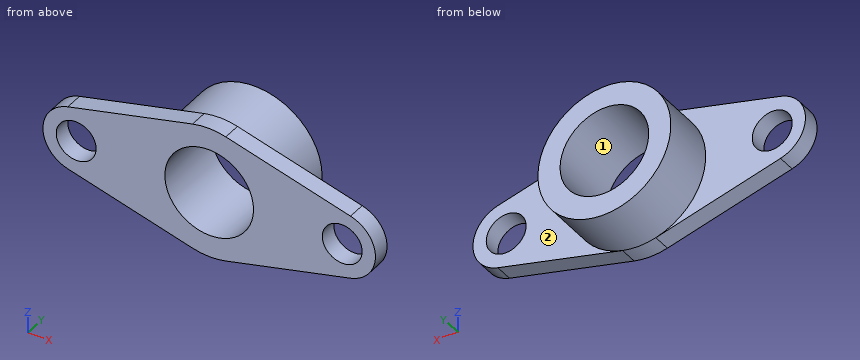
from build123d import *

# Parameters (mm, degrees)
SKETCH2_R           = 2.25
SKETCH2_R_2         = 5
BOSS_EXTRUDE2_DEPTH = 2
SKETCH3_R           = 7.5
SKETCH3_R_2         = 5
BOSS_EXTRUDE3_DEPTH = 6


with BuildPart() as part:
    # Sketch2 → Boss-Extrude2 (new body)
    with BuildSketch(Plane(origin=(0, 0, 0), x_dir=(1, 0, 0), z_dir=(0, 1, 0))):
        with BuildLine():
            Line((-1.875, 7.261843774), (-15.9375, 3.630921887))
            ThreePointArc((-15.9375, 3.630921887), (-18.75, 0), (-15.9375, -3.630921887))
            Line((-15.9375, -3.630921887), (-1.875, -7.261843774))
            ThreePointArc((-1.875, -7.261843774), (0, -7.5), (1.875, -7.261843774))
            Line((1.875, -7.261843774), (15.9375, -3.630921887))
            ThreePointArc((15.9375, -3.630921887), (18.75, 0), (15.9375, 3.630921887))
            Line((15.9375, 3.630921887), (1.875, 7.261843774))
            ThreePointArc((1.875, 7.261843774), (0, 7.5), (-1.875, 7.261843774))
        make_face()
        with Locations((-15, 0)):
            Circle(SKETCH2_R, mode=Mode.SUBTRACT)
        Circle(SKETCH2_R_2, mode=Mode.SUBTRACT)
        with Locations((15, 0)):
            Circle(SKETCH2_R, mode=Mode.SUBTRACT)
    extrude(amount=BOSS_EXTRUDE2_DEPTH)

    # Sketch3 → Boss-Extrude3 (add)
    with BuildSketch(Plane(origin=(0, 2, 0), x_dir=(1, 0, 0), z_dir=(0, 1, 0))):
        Circle(SKETCH3_R)
        Circle(SKETCH3_R_2, mode=Mode.SUBTRACT)
    extrude(amount=BOSS_EXTRUDE3_DEPTH)


solid = part.part
Verification items for the finished model (mm, model axes). Face numbers are marked on the shaded views. Round coordinates to 2 decimals unless told otherwise and drop trailing zeros. Loops run counter-clockwise (first coordinate to the right, second up) from the corner with the lowest first, then second, coordinate; pieces in that order, holes last. Notation, with made-up numbers: (48, 43.25) - (95, 43.25) arc R15 cw to (95, 52.25) - close; hole circle Ø4 at (53.25, -25). An arc over 180 degrees is marked (long way). Use a Markdown table: item, result. Add a question column.
1. Section check A-A, the plane z = 0. Record the boundary of the cut face in (x, y), plus the area to 3 significant figures.
2. Gauge pin test, flat ends, axial feed: pin 1 (2 mm diameter, centred on x = -4.5, y = 4.5, fed in from -Z); pin 2 (2 mm diameter, centred on x = 14, z = -1.5, fed in from +Y). Record the tip position at first contact, or that the pin passes through.
3. Thickness scan on probe 1 along X at (y, z) = (0.75, -1.25); probe 2 along Z at (x, y) = (0, 4.75); probe 3 along X at (y, z) = (7, -3.75). Record the ranges inside material, lowest first. Write a range as [from, to].
4. Release check for a two-part mould opening along X. For the marked faces 1 and 2 record: released by +X, released by -X, zero draft, split by the parting line, or undercut.
5. Section check C-C, the plane x = 0. Record the boundary of the cut face in (y, z).
6. Section check D-D, the plane z = -3. Record the boundary of the cut face in (x, y), plus the area to 3 significant figures.
7. Section check B-B, the plane y = 1.5. Give the number of separate pieces and of enclosed holes in the cut face, plus the area to 3 significant figures.
Checks:
| question | item | result |
|---|---|---|
| 1 | outline | (-18.75, 0) - (-17.25, 0) - (-17.25, 2) - (-18.75, 2) - close; (-12.75, 0) - (-5, 0) - (-5, 8) - (-7.5, 8) - (-7.5, 2) - (-12.75, 2) - close; (5, 0) - (12.75, 0) - (12.75, 2) - (7.5, 2) - (7.5, 8) - (5, 8) - close; (17.25, 0) - (18.75, 0) - (18.75, 2) - (17.25, 2) - close |
| 1 | area | 67.0 mm^2 |
| 2 | pin 1 | stops at z = -6.63 |
| 2 | pin 2 | stops at y = 2 |
| 3 | probe 1 | x = [-18.54, -16.87], [-13.13, -4.84], [4.84, 13.13], [16.87, 18.54] |
| 3 | probe 2 | z = [-7.5, -5], [5, 7.5] |
| 3 | probe 3 | x = [-6.5, -3.31], [3.31, 6.5] |
| 4 | face 1 | undercut |
| 4 | face 2 | zero draft |
| 5 | outline | (0, -7.5) - (8, -7.5) - (8, -5) - (0, -5) - close; (0, 5) - (8, 5) - (8, 7.5) - (0, 7.5) - close |
| 6 | outline | (-17.25, 0) - (-4, 0) - (-4, 8) - (-6.87, 8) - (-6.87, 2) - (-17.25, 2) - close; (4, 0) - (17.25, 0) - (17.25, 2) - (6.87, 2) - (6.87, 8) - (4, 8) - close |
| 6 | area | 87.5 mm^2 |
| 7 | separate pieces | 1 |
| 7 | enclosed holes | 3 |
| 7 | area | 282 mm^2 |
